Part print with two shaded views. Sizes in mm from the minimum x, y, z corner. A direction names the side the tool comes from. Coordinates: 2 decimals unless noted, no trailing zeros. Loops run counter-clockwise (first coordinate to the right, second up) from the corner with the lowest first, then second, coordinate; pieces in that order, holes last. Notation, with made-up numbers: (67.5, -37) -> (111.5, -37) arc R7 cw to (111.5, -30) -> close; hole circle Ø11 at (56.5, 46.25). An arc over 180 degrees is marked (long way). Use one line per item in the form item = value.
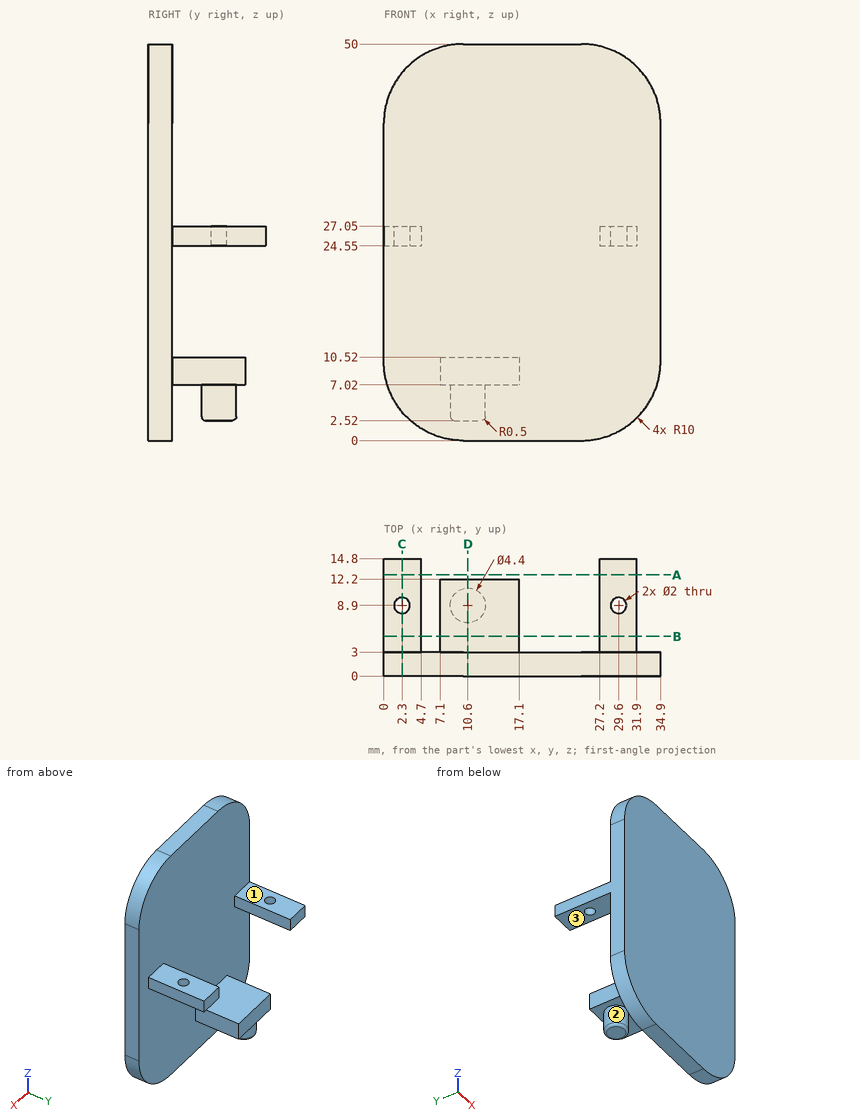
Q1. Band-saw the part on C-C, the plane x = 2.3. Write the cut outline in (y, z).
Result:
outline = (0, 3.62) -> (3, 3.62) -> (3, 24.55) -> (7.9, 24.55) -> (7.9, 27.05) -> (3, 27.05) -> (3, 46.38) -> (0, 46.38) -> close; (9.9, 24.55) -> (14.8, 24.55) -> (14.8, 27.05) -> (9.9, 27.05) -> close
Q2. Which spindle directions (+Z, -Z, +X, -X, +Y, -Y) get a long thin tool onto all of the face, cutting with end or side? Do the marked faces 1, 2 and 3. Say none if no direction does.
Result:
face_1 = +Z, +X, -X, +Y
face_2 = -Z
face_3 = -Z, +X, -X, +Y
Q3. Pin check, flat tips, straight feed: pin 1 Ø2.5 at (x, y) = (30.5, 7.5) entering from -Z; pin 2 Ø0.8 at (y, z) = (10, 25.5) entering from +X; pin 3 Ø3 at (y, z) = (8, 8) entering from -X; pin 4 Ø1.2 at (x, y) = (29.6, 8.9) entering from -Z. Stop position of each tip, or through.
Result:
pin_1 = 24.55
pin_2 = 31.9
pin_3 = 7.1
pin_4 = through
Q4. Band-saw the part on D-D, the plane x = 10.6. Write the cut outline in (y, z), and give its area (3 significant figures).
Result:
outline = (0, 0) -> (3, 0) -> (3, 7.02) -> (6.7, 7.02) -> (6.7, 3.02) arc R0.5 ccw to (7.2, 2.52) -> (10.6, 2.52) arc R0.5 ccw to (11.1, 3.02) -> (11.1, 7.02) -> (12.2, 7.02) -> (12.2, 10.52) -> (3, 10.52) -> (3, 50) -> (0, 50) -> close
area = 202 mm2
Q5. Wall check: line 1 along Z through (x, y) = (11, 8.5); line 2 along Y through (x, z) = (2, 32); line 3 along Z through (x, y) = (9, 5). Give the ranges that are in metal, low to high.
Result:
line_1 = 2.52 to 10.52
line_2 = 0 to 3
line_3 = 7.02 to 10.52
Q6. Band-saw the part on B-B, the plane y = 5. Write the cut outline in (x, z), and give its area (3 significant figures).
Result:
outline = (0, 24.55) -> (4.7, 24.55) -> (4.7, 27.05) -> (0, 27.05) -> close; (7.1, 7.02) -> (17.1, 7.02) -> (17.1, 10.52) -> (7.1, 10.52) -> close; (27.2, 24.55) -> (31.9, 24.55) -> (31.9, 27.05) -> (27.2, 27.05) -> close
area = 58.5 mm2
Q7. Band-saw the part on A-A, the plane y = 12.75. Write the cut outline in (x, z).
Result:
outline = (0, 24.55) -> (4.7, 24.55) -> (4.7, 27.05) -> (0, 27.05) -> close; (27.2, 24.55) -> (31.9, 24.55) -> (31.9, 27.05) -> (27.2, 27.05) -> close
